Input: part model. Units: mm. Frame: model coordinates. A direction names the side the tool comes from. Coordinates: 2 decimals unless noted, no trailing zeros. Order: outer loops, then holes, each group sorted by start corner. A loop starts at its lowest first (then second) coordinate and runs counter-clockwise, first axis right, second up. Notation, with made-up numbers: (-3.75, 84) - (29.25, 84) arc R14 ccw to (29.25, 98) - close; hole circle Ø5 at (84.25, -39.5). An arc over 180 degrees is marked (long way). One line per question, with ' | ' between items.
from build123d import *

# Parameters (mm, degrees)
ESBO_O1_W                = 120
ESBO_O1_H                = 120
ESBO_O1_R                = 2.75
RESSALTO_EXTRUS_O1_DEPTH = 2.5
FILETE1_R                = 15
ESBO_O2_R                = 3.975
RESSALTO_EXTRUS_O2_DEPTH = 22
ESBO_O3_R                = 10
RESSALTO_EXTRUS_O3_DEPTH = 1


with BuildPart() as part:
    # Esboço1 → Ressalto-extrusão1 (new, symmetric)
    with BuildSketch(Plane(origin=(0, 0, 0), x_dir=(1, 0, 0), z_dir=(0, 1, 0))):
        Rectangle(ESBO_O1_W, ESBO_O1_H)
        with Locations(Location((-50.955395397, -50.955395397, 0), (0, 0, 270))):
            Circle(ESBO_O1_R, mode=Mode.SUBTRACT)
        with Locations(Location((-50.955395397, 50.955395397, 0), (0, 0, 270))):
            Circle(ESBO_O1_R, mode=Mode.SUBTRACT)
        with Locations(Location((50.955395397, 50.955395397, 0), (0, 0, 270))):
            Circle(ESBO_O1_R, mode=Mode.SUBTRACT)
        with Locations(Location((50.955395397, -50.955395397, 0), (0, 0, 270))):
            Circle(ESBO_O1_R, mode=Mode.SUBTRACT)
    extrude(amount=RESSALTO_EXTRUS_O1_DEPTH, both=True)

    # Filete1
    filete1_edges = [part.edges().sort_by_distance(p)[0] for p in [
        (-60, 0, 60),
        (-60, 0, -60),
        (60, 0, -60),
        (60, 0, 60),
    ]]
    fillet(filete1_edges, radius=FILETE1_R)

    # Esboço2 → Ressalto-extrusão2 (add)
    with BuildSketch(Plane(origin=(0, 2.5, 0), x_dir=(1, 0, 0), z_dir=(0, 1, 0))):
        with Locations(Location((0, 0, 0), (0, 0, 270))):
            Circle(ESBO_O2_R)
    extrude(amount=RESSALTO_EXTRUS_O2_DEPTH)

    # Esboço3 → Ressalto-extrusão3 (add)
    with BuildSketch(Plane(origin=(0, 2.5, 0), x_dir=(1, 0, 0), z_dir=(0, 1, 0))):
        with Locations(Location((0, 0, 0), (0, 0, 270))):
            Circle(ESBO_O3_R)
    extrude(amount=RESSALTO_EXTRUS_O3_DEPTH)


solid = part.part
Item 1: Access query for faces 1 (the face through (-2.419, 13.853, -3.154)), 2 (the face through (-1, -2.5, -1)). Directions: +Z, -Z, +X, -X, +Y, -Y. A direction counts if a zero-diameter tool reaches every point of the face in a straight line with its end or side. Return the directions, or none.
Data:
face 1: +Y | face 2: +Z, -Z, +X, -X, -Y
Item 2: Section A-A on x = 0. Return the cut outline in (y, z) (3 decimals).
Data:
outline: (-2.5, -60) - (2.5, -60) - (2.5, -10) - (3.5, -10) - (3.5, -3.975) - (24.5, -3.975) - (24.5, 3.975) - (3.5, 3.975) - (3.5, 10) - (2.5, 10) - (2.5, 60) - (-2.5, 60) - close
Item 3: Contact query for flat-ended pins moving along their axis: P1, Ø10, axis at x = -1, y = 6.5, coming from the +Z side; P2, Ø6.5, axis at x = 50.96, z = -50.96, coming from the +Y side; P3, Ø4, axis at x = -5, y = 16, coming from the -Z side; P4, Ø6, axis at x = 25, y = 6.5, coming from the -Z side. Output: stop coordinate, or through.
Data:
P1: z = 60 | P2: y = 2.5 | P3: z = -2.61 | P4: through
Item 4: Section B-B on z = 0. Return the cut outline in (x, y) (3 decimals), and give its area (3 significant figures).
Data:
outline: (-60, -2.5) - (60, -2.5) - (60, 2.5) - (10, 2.5) - (10, 3.5) - (3.975, 3.5) - (3.975, 24.5) - (-3.975, 24.5) - (-3.975, 3.5) - (-10, 3.5) - (-10, 2.5) - (-60, 2.5) - close | area: 787 mm^2
Item 5: Ray query, line 1 (Y direction, x = 39, z = 36); line 2 (X direction, y = 15.75, z = 0.5); line 3 (X direction, y = 0.25, z = -55). Return the intervals inside material, ascending.
Data:
line 1: -2.5 to 2.5 | line 2: -3.94 to 3.94 | line 3: -56.18 to 56.18
Item 6: Section D-D on x = -12.5. Return the cut outline in (y, z), and give its area (3 significant figures).
Data:
outline: (-2.5, -60) - (2.5, -60) - (2.5, 60) - (-2.5, 60) - close | area: 600 mm^2
Item 7: Section C-C on y = 19.5. Return the cut outline in (x, z) (3 decimals), and give its area (3 significant figures).
Data:
outline: circle Ø7.95 at (0, 0) | area: 49.6 mm^2
Item 8: Draft query along X for faces 3 (the face through (-55.72, 0.04, 55.49)), 4 (the face through (-9.76, 2.99, -2.17)), 5 (the face through (-50.13, -0.04, 53.58)). Return one class per face: released by +X, released by -X, zero draft, split by the parting line, or undercut.
Data:
face 3: released by -X | face 4: split by the parting line | face 5: undercut
